```python
from build123d import *

# Parameters (mm, degrees)
F0_W      = 120
F0_H      = 120
F1_DEPTH  = 3
F2_W      = 15
F2_H      = 15
F3_DEPTH  = 20
F4_W      = 10
F4_H      = 10
F5_DEPTH  = 10
F6_W      = 20.4
F6_H      = 25
F7_DEPTH  = 33
F8_W      = 16.4
F8_H      = 21
F9_DEPTH  = 30
F10_W     = 20.4
F10_H     = 10
F11_DEPTH = 30
F12_W     = 10
F12_H     = 25
F13_DEPTH = 30


with BuildPart() as f1:
    # F0 (on Top) → F1 (new body)
    with BuildSketch(Plane.XY):
        Rectangle(F0_W, F0_H)
    extrude(amount=F1_DEPTH)

    # F2 (on face) → F3 (join)
    with BuildSketch(Plane.XY.offset(3)):
        with Locations((-52.5, 52.5)):
            Rectangle(F2_W, F2_H)
        with Locations((-52.5, -52.5)):
            Rectangle(F2_W, F2_H)
        with Locations((52.5, -52.5)):
            Rectangle(F2_W, F2_H)
        with Locations((52.5, 52.5)):
            Rectangle(F2_W, F2_H)
    extrude(amount=F3_DEPTH)

    # F4 (on face) → F5 (join)
    with BuildSketch(Plane.XY.offset(23)):
        with Locations((-52.5, -52.5)):
            Rectangle(F4_W, F4_H)
        with Locations((52.5, -52.5)):
            Rectangle(F4_W, F4_H)
        with Locations((-52.5, 52.5)):
            Rectangle(F4_W, F4_H)
        with Locations((52.5, 52.5)):
            Rectangle(F4_W, F4_H)
    extrude(amount=F5_DEPTH)

    # F6 (on Top) → F7 (join)
    with BuildSketch(Plane.XY):
        Rectangle(F6_W, F6_H)
    extrude(amount=F7_DEPTH)

    # F8 (on face) → F9 (cut)
    with BuildSketch(Plane.XY.offset(33)):
        Rectangle(F8_W, F8_H)
    extrude(amount=-F9_DEPTH, mode=Mode.SUBTRACT)

    # F10 (on face) → F11 (cut)
    with BuildSketch(Plane.XY.offset(33)):
        Rectangle(F10_W, F10_H)
    extrude(amount=-F11_DEPTH, mode=Mode.SUBTRACT)

    # F12 (on face) → F13 (cut)
    with BuildSketch(Plane.XY.offset(33)):
        Rectangle(F12_W, F12_H)
    extrude(amount=-F13_DEPTH, mode=Mode.SUBTRACT)


solid = f1.part
```
Design review of the part built by this model. Coordinates are the model's own, in mm. A direction names the side the tool comes from. Round coordinates to 2 decimals unless told otherwise and drop trailing zeros. Write each loop counter-clockwise with the first axis right and the second up, starting at its lowest first coordinate (ties: lowest second). Pieces come first, ordered by that corner, then holes.
Item 1: We need section B-B on z = 29. State how many separate pieces and enclosed holes the cut face has, and give its area (3 significant figures).
Item 2: For faces 1 (the flat face through (10.2, -9, 18)), 2 (the flat face through (52, -45, 13)), 3 (the flat face through (-53, -57.5, 28)), 4 (the flat face through (-57.5, -53, 28)), 5 (the flat face through (7, 10.5, 18)), list the 3-axis set-ups (+Z, -Z, +X, -X, +Y, -Y) from which the entire face can be reached by the end or side of a thin tool; tool diameter is ignored.
Item 3: We need section C-C on y = 41. Write out the cut boundary in (x, z).
Item 4: For probe 1 along X at (y, z) = (-52, 25); probe 2 along Y at (x, z) = (53, 18); probe 3 along X at (y, z) = (8, 22), list the stretches that pass through material, from the lowest coordinate up.
Item 5: Clearance check with flat-ended pins moving along their axes: pin 1 Ø0.6 at (x, z) = (9, 18.5) entering from +Y; pin 2 Ø5.5 at (x, z) = (-7, 13) entering from -Y; pin 3 Ø2 at (y, z) = (11, 14) entering from +X. State where each tip first meets the part, or that it passes through.
Item 6: We need section A-A on x = 49. Write out the cut boundary in (y, z), and give its area (3 significant figures).
Returned:
1. separate pieces: 8
1. enclosed holes: 0
1. area: 486 mm2
2. face 1: +Z, +X, +Y, -Y
2. face 2: +Z, +X, -X
2. face 3: +Z, +X, -X, -Y
2. face 4: +Z, -X, +Y, -Y
2. face 5: +Z
3. outline: (-60, 0) - (60, 0) - (60, 3) - (-60, 3) - close
4. probe 1: x = -57.5 to -47.5, 47.5 to 57.5
4. probe 2: y = -60 to -45, 45 to 60
4. probe 3: x = -10.2 to -8.2, 8.2 to 10.2
5. pin 1: stops at y = 12.5
5. pin 2: stops at y = -12.5
5. pin 3: stops at x = 10.2
6. outline: (-60, 0) - (60, 0) - (60, 23) - (57.5, 23) - (57.5, 33) - (47.5, 33) - (47.5, 23) - (45, 23) - (45, 3) - (-45, 3) - (-45, 23) - (-47.5, 23) - (-47.5, 33) - (-57.5, 33) - (-57.5, 23) - (-60, 23) - close
6. area: 1,160 mm2
